Autodesk Inventor part; units mm, degrees
ref_plane "YZ Plane" through (0, 0, 0) normal (1, 0, 0) x (0, 1, 0)
ref_plane "XZ Plane" through (0, 0, 0) normal (0, 1, 0) x (-1, 0, 0)
ref_plane "XY Plane" through (0, 0, 0) normal (0, 0, 1) x (1, 0, 0)
sketch "Sketch1" plane through (0, 0, 0) normal (0, 0, 1) x (1, 0, 0)
  line L0 (-4, 11.7077) -> (6, 1.7077)
  line L1 (-4, 11.7077) -> (-5, 11.7077)
  arc A0 (-5, 11.7077) -> (-6, 10.7077) centre (-5, 10.7077) ccw
  line L2 (-6, 10.7077) -> (-6, -9.2784)
  arc A1 (-6, -9.2784) -> (-4.6842, -10.2272) centre (-5, -9.2784) ccw
  arc A2 (3.1184, -11.5061) -> (-4.6842, -10.2272) centre (-2, -18.2923) ccw
  arc A3 (3.1184, -11.5061) -> (3.7205, -11.7077) centre (3.7205, -10.7077) ccw
  line L3 (3.7205, -11.7077) -> (5, -11.7077)
  arc A4 (5, -11.7077) -> (6, -10.7077) centre (5, -10.7077) ccw
  line L4 (6, -10.7077) -> (6, 1.7077)
  arc A5 (5, -36.8923) -> (6, -35.8923) centre (5, -35.8923) ccw
  line L5 (6, -35.8923) -> (6, -27.7923)
  arc A6 (6, -27.7923) -> (5, -26.7923) centre (5, -27.7923) ccw
  line L6 (5, -26.7923) -> (-1.4303, -26.7923)
  arc A7 (-1.4303, -26.7923) -> (-2.3324, -28.2239) centre (-1.4303, -27.7923) ccw
  arc A8 (-2.2902, -35.4712) -> (-2.3324, -28.2239) centre (-10, -31.8923) ccw
  arc A9 (-2.2902, -35.4712) -> (-1.3832, -36.8923) centre (-1.3832, -35.8923) ccw
  line L7 (-1.3832, -36.8923) -> (5, -36.8923)
  line L8 (6, -53.1923) -> (6, -35.8923)
  line L9 (6, -27.7923) -> (6, -10.7077)
  line L10 (-5, 11.7077) -> (-20, 11.7077)
  line L11 (-20, 11.7077) -> (-35, 11.7077)
  line L12 (6, -68.1923) -> (6, -53.1923)
  line L13 (-35, 306.8077) -> (-35, -53.1923)
  line L14 (-35, -68.1923) -> (-35, -53.1923)
  line L15 (-20, -68.1923) -> (-35, -68.1923)
  line L16 (480, -68.1923) -> (-20, -68.1923)
  circle A10 centre (2, -2.1923) radius 1.4
  circle A11 centre (2, -32.1923) radius 1.4
  circle A12 centre (2, -2.1923) radius 1.75
  circle A13 centre (2, -32.1923) radius 1.75
  circle A14 centre (-10, -31.9923) radius 2.5
  circle A15 centre (-2, -18.3923) radius 2.5
  point P0 (0, 0)
  dimension "d18" = 3.5
extrude "Extrusion1" add sketch "Sketch1" along normal blind 3 contours L0 L4 A4 L3 A3 A2 A1 L2 A0 L1 | A0 L2 A1 A2 A3 L3 A4 L9 A6 L6 A7 A8 A9 L7 A5 L8 L12 L16 L15 L14 L13 L11 L10 | L5 A5 L7 A9 A8 A7 L6 A6
sketch "Sketch2" plane through (0, 0, 0) normal (0, 0, -1) x (-1, 0, 0)
  line L0 (-6, -68.1923) -> (-6, 1.7077)
  line L1 (35, -68.1923) -> (-6, -68.1923)
  line L2 (35, 11.7077) -> (35, -68.1923)
  line L3 (4, 11.7077) -> (35, 11.7077)
  line L4 (-6, 1.7077) -> (4, 11.7077)
  line L5 (20, 11.7077) -> (20, -53.1923)
  line L6 (20, -53.1923) -> (-6, -53.1923)
  line L7 (-6, -68.1923) -> (-6, 1.7077)
  point P0 (0, 0)
  point P1 (7, -53.1923)
  dimension "d2" = 15
  dimension "d3" = 15
extrude "Extrusion2" add sketch "Sketch2" along normal blind 3 contours L0 L6 L5 L3 L2 L1
sketch "Sketch3" plane through (0, 0, 3) normal (0, 0, 1) x (1, 0, 0)
  line L0 (6, -68.1923) -> (6, 1.7077)
  line L1 (6, 1.7077) -> (-4, 11.7077)
  line L2 (-4, 11.7077) -> (-35, 11.7077)
  line L3 (-35, 11.7077) -> (-35, -68.1923)
  line L4 (-35, -68.1923) -> (6, -68.1923)
  circle A0 centre (2, -2.2923) radius 1.4
  circle A1 centre (2, -32.2923) radius 1.4
  point P0 (0, 0)
  point P1 (-27.5, -3.2923)
  point P2 (-27.5, -43.2923)
  point P3 (-4, -60.6923)
  dimension "d6" = 7.5
  dimension "d7" = 10
  dimension "d8" = 7.5
  dimension "d9" = 15
  dimension "d10" = 40
hole "Hole1" at (-27.5, -3.2923, 3) at (-27.5, -43.2923, 3) at (-4, -60.6923, 3) direction (0, 0, -1) diameter 3.6 end through all counterbore diameter 6.5 counterbore depth 3.4
properties part number "Alpha Idler Top" material "ABS Plastic"
Verification items for the finished model (mm, model axes). A direction names the side the tool comes from. Give positions to 0.01 mm unless a question says otherwise; leave off trailing zeros. Loops run counter-clockwise (first coordinate to the right, second up) from the corner with the lowest first, then second, coordinate; pieces in that order, holes last.
1. Set-up check for faces 1 (the flat face through (6, -41, 1)), 2 (the flat face through (-2.6, -62.1, -0.4)), 3 (the flat face through (-7, -20, 0)): record each of +Z, -Z, +X, -X, +Y, -Y from which the full face is reachable in a straight line by a thin tool's end or side.
2. Section check C-C, the plane z = -1.5. Enter the section's corners in (x, y).
3. Thickness scan on line 1 (Y direction, x = -27.5, z = 1.9); line 2 (Y direction, x = -10, z = 2.1); line 3 (Y direction, x = -4, z = -2.3). Record the ranges inside material, lowest first.
4. Section check D-D, the plane y = -43.5. Enter the section's corners in (x, z), then the cut area to 3 significant figures.
5. Section check A-A, the plane x = -10. Enter the section's corners in (y, z).
6. Go/stop test with flat-tipped pins: pin 1 Ø4 at (x, y) = (-27.5, -43.29) entering from +Z; pin 2 Ø8 at (x, y) = (-3.5, -16) entering from -Z; pin 3 Ø0.9 at (y, z) = (-5, -1) entering from +X; pin 4 Ø2 at (x, y) = (-27.5, -43.29) entering from +Z. Record where each tip stops, or that it passes through.
7. Section check B-B, the plane x = -27.5. Enter the section's corners in (y, z), then the cut area to 3 significant figures.
Geometry says:
1. face 1: +Z, -Z, +X, +Y, -Y
1. face 2: +Z
1. face 3: -Z, +X, +Y
2. outline: (-35, -68.19) - (6, -68.19) - (6, -53.19) - (-20, -53.19) - (-20, 11.71) - (-35, 11.71) - close; hole circle Ø3.6 at (-27.5, -43.29); hole circle Ø3.6 at (-27.5, -3.29); hole circle Ø3.6 at (-4, -60.69)
3. line 1: y = -68.19 to -46.54, -40.04 to -6.54, -0.04 to 11.71
3. line 2: y = -68.19 to -34.49, -29.49 to 11.71
3. line 3: y = -68.19 to -62.49, -58.89 to -53.19
4. outline: (-35, -3) - (-29.29, -3) - (-29.29, -0.4) - (-30.74, -0.4) - (-30.74, 3) - (-35, 3) - close; (-25.71, -3) - (-20, -3) - (-20, 0) - (6, 0) - (6, 3) - (-24.26, 3) - (-24.26, -0.4) - (-25.71, -0.4) - close
4. area: 137 mm2
5. outline: (-68.19, -3) - (-53.19, -3) - (-53.19, 0) - (-34.49, 0) - (-34.49, 3) - (-68.19, 3) - close; (-29.49, 0) - (11.71, 0) - (11.71, 3) - (-29.49, 3) - close
6. pin 1: stops at z = -0.4
6. pin 2: stops at z = 0
6. pin 3: stops at x = -20
6. pin 4: passes through
7. outline: (-68.19, -3) - (-45.09, -3) - (-45.09, -0.4) - (-46.54, -0.4) - (-46.54, 3) - (-68.19, 3) - close; (-41.49, -3) - (-5.09, -3) - (-5.09, -0.4) - (-6.54, -0.4) - (-6.54, 3) - (-40.04, 3) - (-40.04, -0.4) - (-41.49, -0.4) - close; (-1.49, -3) - (11.71, -3) - (11.71, 3) - (-0.04, 3) - (-0.04, -0.4) - (-1.49, -0.4) - close
7. area: 416 mm2
